Source: CAD feature listing. Evaluate the final solid. Frame: model axes, mm. Face numbers are marked on the shaded views. Round coordinates to 2 decimals unless told otherwise and drop trailing zeros. Write each loop counter-clockwise with the first axis right and the second up, starting at its lowest first coordinate (ties: lowest second). Pieces come first, ordered by that corner, then holes. Notation, with made-up numbers: M -32,-3.75 L 3,-3.75 A21 ccw 3,28.25 Z; hole C -20,-22 d7. An arc over 180 degrees is marked long. Answer in a Markdown table with one row per item.
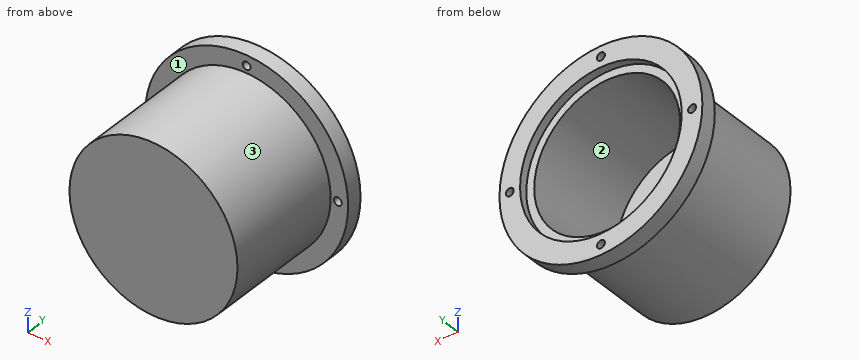
from build123d import *

# Parameters (mm, degrees)
SKETCH1_R           = 53
BOSS_EXTRUDE1_DEPTH = 75
SKETCH2_R           = 64
BOSS_EXTRUDE2_DEPTH = 10
SKETCH3_R           = 51
CUT_EXTRUDE1_DEPTH  = 5
SKETCH5_R           = 46
CUT_EXTRUDE2_DEPTH  = 66
SKETCH6_R           = 2.5
CUT_EXTRUDE3_DEPTH  = 66


with BuildPart() as part:
    # Sketch1 → Boss-Extrude1 (new body)
    with BuildSketch(Plane(origin=(0, 0, 0), x_dir=(1, 0, 0), z_dir=(0, 1, 0))):
        Circle(SKETCH1_R)
    extrude(amount=BOSS_EXTRUDE1_DEPTH)

    # Sketch2 → Boss-Extrude2 (add)
    with BuildSketch(Plane(origin=(0, 75, 0), x_dir=(1, 0, 0), z_dir=(0, 1, 0))):
        Circle(SKETCH2_R)
    extrude(amount=BOSS_EXTRUDE2_DEPTH)

    # Sketch3 → Cut-Extrude1 (cut)
    with BuildSketch(Plane(origin=(0, 85, 0), x_dir=(1, 0, 0), z_dir=(0, 1, 0))):
        Circle(SKETCH3_R)
    extrude(amount=-CUT_EXTRUDE1_DEPTH, mode=Mode.SUBTRACT)

    # Sketch5 → Cut-Extrude2 (cut)
    with BuildSketch(Plane(origin=(0, 80, 0), x_dir=(1, 0, 0), z_dir=(0, 1, 0))):
        Circle(SKETCH5_R)
    extrude(amount=-CUT_EXTRUDE2_DEPTH, mode=Mode.SUBTRACT)

    # Sketch6 → Cut-Extrude3 (cut)
    with BuildSketch(Plane(origin=(0, 85, 0), x_dir=(1, 0, 0), z_dir=(0, 1, 0))):
        with Locations((-57.5, 0)):
            Circle(SKETCH6_R)
        with Locations((0, 57.5)):
            Circle(SKETCH6_R)
        with Locations((57.5, 0)):
            Circle(SKETCH6_R)
        with Locations((0, -57.5)):
            Circle(SKETCH6_R)
    extrude(amount=-CUT_EXTRUDE3_DEPTH, mode=Mode.SUBTRACT)


solid = part.part
Q1. Section D-D (z = -57.5). Return loops of the section in (x, y), and give its area (3 significant figures).
Solutions:
| item | result |
|---|---|
| outline | M -28.1,75 L -2.5,75 L -2.5,85 L -28.1,85 Z; M 2.5,75 L 28.1,75 L 28.1,85 L 2.5,85 Z |
| area | 512 mm2 |
Q2. Section A-A (z = 0). Return loops of the section in (x, y), and give its area (3 significant figures).
Solutions:
| item | result |
|---|---|
| outline | M -64,75 L -60,75 L -60,85 L -64,85 Z; M -55,75 L -53,75 L -53,0 L 53,0 L 53,75 L 55,75 L 55,85 L 51,85 L 51,80 L 46,80 L 46,14 L -46,14 L -46,80 L -51,80 L -51,85 L -55,85 Z; M 60,75 L 64,75 L 64,85 L 60,85 Z |
| area | 2,550 mm2 |
Q3. Pull-direction query (Z, two-part tool) for the marked faces 1, 2 and 3; classes: pulls with the +Z half, pulls with the -Z half, needs draft (parallel to the pull), parting line crosses it, or undercut.
Solutions:
| item | result |
|---|---|
| face 1 | needs draft |
| face 2 | undercut |
| face 3 | parting line crosses it |
Q4. Section B-B (x = 0). Return loops of the section in (y, z), and give its area (3 significant figures).
Solutions:
| item | result |
|---|---|
| outline | M 0,-53 L 75,-53 L 75,-55 L 85,-55 L 85,-51 L 80,-51 L 80,-46 L 14,-46 L 14,46 L 80,46 L 80,51 L 85,51 L 85,55 L 75,55 L 75,53 L 0,53 Z; M 75,-64 L 85,-64 L 85,-60 L 75,-60 Z; M 75,60 L 85,60 L 85,64 L 75,64 Z |
| area | 2,550 mm2 |
Q5. Section C-C (x = -57.5). Return loops of the section in (y, z).
Solutions:
| item | result |
|---|---|
| outline | M 75,-28.1 L 85,-28.1 L 85,-2.5 L 75,-2.5 Z; M 75,2.5 L 85,2.5 L 85,28.1 L 75,28.1 Z |
Q6. Material intervals for probe 1 along Z at (x, y) = (0, 81.5); probe 2 along Z at (x, y) = (0, 77.5), sorted ascending.
Solutions:
| item | result |
|---|---|
| probe 1 | z = -64 to -60, -55 to -51, 51 to 55, 60 to 64 |
| probe 2 | z = -64 to -60, -55 to -46, 46 to 55, 60 to 64 |
Q7. Contact query for flat-ended pins moving along their axis: pin 1 Ø4 at (x, z) = (-19, -2) entering from -Y; pin 2 Ø4.5 at (x, z) = (-57.5, 0) entering from -Y; pin 3 Ø12 at (y, z) = (22, 27) entering from -X; pin 4 Ø5 at (x, y) = (49, 44.5) entering from +Z. Output: stop coordinate, or through.
Solutions:
| item | result |
|---|---|
| pin 1 | stops at y = 0 |
| pin 2 | passes through |
| pin 3 | stops at x = -48.66 |
| pin 4 | stops at z = 25.43 |
